```python
from build123d import *

# Parameters (mm, degrees)
SKETCH1_R              = 17.5
BASE_EXTRUDE_DEPTH     = 8
PROCESS_BENDS2_START   = 80
PROCESS_BENDS2_DEPTH   = 107
PROCESS_BENDS2_2_DEPTH = 107
PROCESS_BENDS2_START_2 = -200
PROCESS_BENDS2_3_DEPTH = 34.194961468


with BuildPart() as part:
    # Sketch1 → Base-Extrude (new body)
    with BuildSketch(Plane.XY):
        with BuildLine():
            Line((-24.35045716, -31.734133612), (32.213121298, -75.1368939))
            ThreePointArc((32.213121298, -75.1368939), (41.442716862, -84.366489464), (47.969026473, -95.670389296))
            Line((47.969026473, -95.670389296), (76.193976626, -163.811446751))
            ThreePointArc((76.193976626, -163.811446751), (79.03926402, -173.191102268), (80, -182.945618369))
            Line((80, -182.945618369), (80, -330))
            ThreePointArc((80, -330), (80.878679656, -332.121320344), (83, -333))
            Line((83, -333), (184, -333))
            ThreePointArc((184, -333), (186.121320344, -332.121320344), (187, -330))
            Line((187, -330), (187, -181))
            ThreePointArc((187, -181), (188.464466094, -177.464466094), (192, -176))
            Line((192, -176), (217, -176))
            ThreePointArc((217, -176), (219.121320344, -175.121320344), (220, -173))
            Line((220, -173), (220, -164.288637004))
            ThreePointArc((220, -164.288637004), (218.128933039, -157.033906323), (212.9825177, -151.589053894))
            Line((212.9825177, -151.589053894), (147.666248084, -110.53351106))
            ThreePointArc((147.666248084, -110.53351106), (140.248070405, -105.389440946), (133.324011991, -99.597357342))
            Line((133.324011991, -99.597357342), (39.541737093, -13.661735283))
            ThreePointArc((39.541737093, -13.661735283), (36.185639292, -8.978306226), (35, -3.339852568))
            Line((35, -3.339852568), (35, 27.261127274))
            ThreePointArc((35, 27.261127274), (34.942355841, 27.84639824), (34.771638598, 28.409177571))
            Line((34.771638598, 28.409177571), (25.767102684, 50.148050297))
            ThreePointArc((25.767102684, 50.148050297), (24.662174785, 51.494408837), (22.995464086, 52))
            Line((22.995464086, 52), (-37, 52))
            ThreePointArc((-37, 52), (-39.121320344, 51.121320344), (-40, 49))
            Line((-40, 49), (-40, 0))
            ThreePointArc((-40, 0), (-35.874909661, -17.691547609), (-24.35045716, -31.734133612))
        make_face()
        Circle(SKETCH1_R, mode=Mode.SUBTRACT)
    extrude(amount=-BASE_EXTRUDE_DEPTH)

    # Process-Bends2: read off the stored shape, not the designer's step
    # Process-Bends2 outline → Process-Bends2 (cut)
    with BuildSketch(Plane.YZ.offset(PROCESS_BENDS2_START)):
        with BuildLine():
            ThreePointArc((-197.729039967, -8), (-208.312045211, -5.922962794), (-217.324957909, 0))
            Line((-217.324957909, 0), (-333, 0))
            Line((-333, 0), (-333, -8))
            Line((-333, -8), (-197.729039967, -8))
        make_face()
    extrude(amount=PROCESS_BENDS2_DEPTH, mode=Mode.SUBTRACT)

    # Process-Bends2 2 outline → Process-Bends2 2 (add)
    with BuildSketch(Plane.YZ.offset(PROCESS_BENDS2_START)):
        with BuildLine():
            Line((-215.855195707, 11.547634765), (-261.806073579, 110.089610364))
            Line((-261.806073579, 110.089610364), (-269.056535875, 106.70866427))
            Line((-269.056535875, 106.70866427), (-223.105658004, 8.166688671))
            ThreePointArc((-223.105658004, 8.166688671), (-220.583053817, 3.823039502), (-217.324957909, 0))
            Line((-217.324957909, 0), (-197.729039967, 0))
            ThreePointArc((-197.729039967, 0), (-208.475032134, 3.132171084), (-215.855195707, 11.547634765))
        make_face()
    extrude(amount=PROCESS_BENDS2_2_DEPTH)

    # Process-Bends2 3 outline → Process-Bends2 3 (cut)
    with BuildSketch(Plane(origin=(0, 0, 0), x_dir=(1, 0, 0), z_dir=(0, 0.9063077870366512, 0.42261826174069705)).offset(PROCESS_BENDS2_START_2)):
        with BuildLine():
            Line((80, -210.419098874), (83, -210.419098874))
            ThreePointArc((83, -210.419098874), (80.878679657, -209.540419218), (80, -207.419098874))
            Line((80, -207.419098874), (80, -210.419098874))
        make_face()
        with BuildLine():
            ThreePointArc((187, -207.419098874), (186.121320343, -209.540419218), (184, -210.419098874))
            Line((184, -210.419098874), (187, -210.419098874))
            Line((187, -210.419098874), (187, -207.419098874))
        make_face()
    extrude(amount=PROCESS_BENDS2_3_DEPTH, mode=Mode.SUBTRACT)


solid = part.part
```
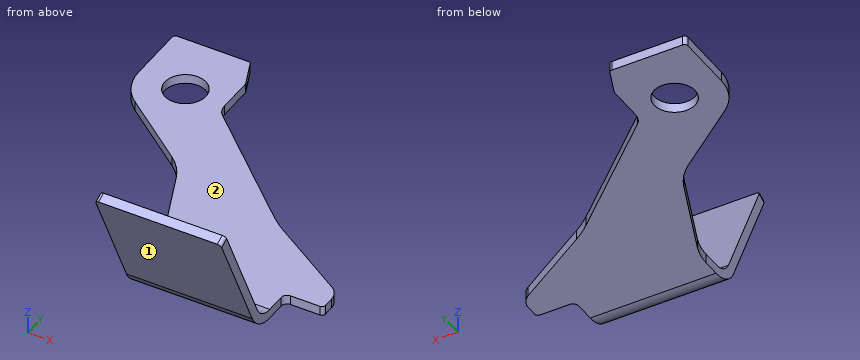
Can you work these out from the model? Positions are in its coordinate system, mm. Face numbers are marked on the shaded views. A direction names the side the tool comes from. Round coordinates to 2 decimals unless told otherwise and drop trailing zeros. Order: outer loops, then holes, each group sorted by start corner. A loop starts at its lowest first (then second) coordinate and runs counter-clockwise, first axis right, second up. Notation, with made-up numbers: (27, -36.5) -> (55, -36.5) arc R32 cw to (55, 2.5) -> close; hole circle Ø4 at (2.25, 57.25). An arc over 180 degrees is marked (long way). Return JSON: item names as keys, results as strings. Group by question number.
1. I need wall thicknesses on line 1 (Z direction, x = 165, y = -136); line 2 (Y direction, x = 0, z = -6); line 3 (X direction, y = 24, z = -2.5). Which ranges of each line are inside material? Lowest first, please. Write a range as [from, to].
2. If we section it at D-D, the plane z = 30: Write out the boundary of the cut face in (x, y).
3. Which directions (+Z, -Z, +X, -X, +Y, -Y) give clear straight access to the entire face, cutting with the end or side of a thin tool? Please do the marked faces 1 and 2.
4. If we section it at B-B, the plane x = 161.5: Write out the boundary of the cut face in (y, z), then the cut area to 3 significant figures.
5. Will these pins go through, and if not, where does the flat tip stop? pin 1 (2 mm diameter, centred on x = 159.5, z = 6.5, fed in from +Y); pin 2 (21 mm diameter, centred on x = 0, y = 0, fed in from -Z); pin 3 (2.5 mm diameter, centred on y = 16.5, z = -3, fed in from +X); pin 4 (12 mm diameter, centred on x = 111.5, z = 93, fed in from -Y).
6. If we section it at A-A, the plane x = 0: Write out the boundary of the cut face in (y, z), then the cut area to 3 significant figures.
7. If we section it at C-C, the plane y = -232.5: Write out the boundary of the cut face in (x, z).
Output values:
{
 "1": {"line 1": "[-8, 0]", "line 2": "[-50.42, -17.5], [17.5, 52]", "line 3": "[-40, 35]"},
 "2": {"outline": "(80, -233.29) -> (187, -233.29) -> (187, -224.46) -> (80, -224.46) -> close"},
 "3": {"face 1": "-Z, +X, -X, -Y", "face 2": "+Z, +X, -X, +Y"},
 "4": {"outline": "(-269.06, 106.71) -> (-223.11, 8.17) arc R28 ccw to (-197.73, -8) -> (-119.23, -8) -> (-119.23, 0) -> (-197.73, 0) arc R20 cw to (-215.86, 11.55) -> (-261.81, 110.09) -> close", "area": "1,720 mm²"},
 "5": {"pin 1": "y = -211.5", "pin 2": "through", "pin 3": "x = 35", "pin 4": "y = -265.46"},
 "6": {"outline": "(-50.42, -8) -> (-17.5, -8) -> (-17.5, 0) -> (-50.42, 0) -> close; (17.5, -8) -> (52, -8) -> (52, 0) -> (17.5, 0) -> close", "area": "539 mm²"},
 "7": {"outline": "(80, 28.31) -> (187, 28.31) -> (187, 47.24) -> (80, 47.24) -> close"}
}
